Work out the finished part from the listing and answer in its coordinate system (mm). Round coordinates to 2 decimals unless told otherwise and drop trailing zeros. Order: outer loops, then holes, each group sorted by start corner. A loop starts at its lowest first (then second) coordinate and runs counter-clockwise, first axis right, second up. Notation, with made-up numbers: M -9,88 L 10,88 A30 cw 10,114 Z; hole C 32,-32.75 d4. An arc over 180 degrees is marked long. Return JSON: item names as keys, results as strings.
from build123d import *

# Parameters (mm, degrees)
SKETCH1_R           = 2.25
SKETCH1_R_2         = 2.5
SKETCH1_W           = 86
SKETCH1_H           = 86
BOSS_EXTRUDE1_DEPTH = 1
FILLET1_R           = 5
FILLET2_R           = 10


with BuildPart() as part:
    # Sketch1 → Boss-Extrude1 (new body)
    with BuildSketch(Plane(origin=(0, 0, 0), x_dir=(1, 0, 0), z_dir=(0, 1, 0))):
        Polygon((-70, -157.5), (447.5, -157.5), (447.5, -92.5), (82.5, -92.5), (82.5, 92.5), (447.5, 92.5), (447.5, 157.5), (-70, 157.5), align=None)
        with Locations(Location((-62.5, 100, 0), (0, 0, 270))):
            Circle(SKETCH1_R, mode=Mode.SUBTRACT)
        with Locations(Location((-62.5, -100, 0), (0, 0, 270))):
            Circle(SKETCH1_R, mode=Mode.SUBTRACT)
        with Locations(Location((-62.5, 150, 0), (0, 0, 270))):
            Circle(SKETCH1_R, mode=Mode.SUBTRACT)
        with Locations(Location((-62.5, -150, 0), (0, 0, 270))):
            Circle(SKETCH1_R, mode=Mode.SUBTRACT)
        with Locations(Location((62.5, -100, 0), (0, 0, 270))):
            Circle(SKETCH1_R, mode=Mode.SUBTRACT)
        with Locations(Location((62.5, -150, 0), (0, 0, 270))):
            Circle(SKETCH1_R, mode=Mode.SUBTRACT)
        with Locations(Location((62.5, 100, 0), (0, 0, 270))):
            Circle(SKETCH1_R, mode=Mode.SUBTRACT)
        with Locations(Location((62.5, 150, 0), (0, 0, 270))):
            Circle(SKETCH1_R, mode=Mode.SUBTRACT)
        with Locations(Location((187.5, -100, 0), (0, 0, 270))):
            Circle(SKETCH1_R, mode=Mode.SUBTRACT)
        with Locations(Location((187.5, -150, 0), (0, 0, 270))):
            Circle(SKETCH1_R, mode=Mode.SUBTRACT)
        with Locations(Location((187.5, 100, 0), (0, 0, 270))):
            Circle(SKETCH1_R, mode=Mode.SUBTRACT)
        with Locations(Location((187.5, 150, 0), (0, 0, 270))):
            Circle(SKETCH1_R, mode=Mode.SUBTRACT)
        with Locations(Location((312.5, -100, 0), (0, 0, 270))):
            Circle(SKETCH1_R, mode=Mode.SUBTRACT)
        with Locations(Location((312.5, -150, 0), (0, 0, 270))):
            Circle(SKETCH1_R, mode=Mode.SUBTRACT)
        with Locations(Location((312.5, 100, 0), (0, 0, 270))):
            Circle(SKETCH1_R, mode=Mode.SUBTRACT)
        with Locations(Location((312.5, 150, 0), (0, 0, 270))):
            Circle(SKETCH1_R, mode=Mode.SUBTRACT)
        with Locations(Location((437.5, -100, 0), (0, 0, 270))):
            Circle(SKETCH1_R, mode=Mode.SUBTRACT)
        with Locations(Location((437.5, -150, 0), (0, 0, 270))):
            Circle(SKETCH1_R, mode=Mode.SUBTRACT)
        with Locations(Location((437.5, 100, 0), (0, 0, 270))):
            Circle(SKETCH1_R, mode=Mode.SUBTRACT)
        with Locations(Location((437.5, 150, 0), (0, 0, 270))):
            Circle(SKETCH1_R, mode=Mode.SUBTRACT)
        with Locations(Location((-43, -73, 0), (0, 0, 270))):
            Circle(SKETCH1_R_2, mode=Mode.SUBTRACT)
        with Locations(Location((43, -73, 0), (0, 0, 270))):
            Circle(SKETCH1_R_2, mode=Mode.SUBTRACT)
        with Locations(Location((-43, 73, 0), (0, 0, 270))):
            Circle(SKETCH1_R_2, mode=Mode.SUBTRACT)
        with Locations(Location((43, 73, 0), (0, 0, 270))):
            Circle(SKETCH1_R_2, mode=Mode.SUBTRACT)
        with Locations(Location((262.5, 150, 0), (0, 0, 270))):
            Circle(SKETCH1_R, mode=Mode.SUBTRACT)
        with Locations(Location((262.5, 100, 0), (0, 0, 270))):
            Circle(SKETCH1_R, mode=Mode.SUBTRACT)
        with Locations(Location((262.5, -100, 0), (0, 0, 270))):
            Circle(SKETCH1_R, mode=Mode.SUBTRACT)
        with Locations(Location((262.5, -150, 0), (0, 0, 270))):
            Circle(SKETCH1_R, mode=Mode.SUBTRACT)
        Rectangle(SKETCH1_W, SKETCH1_H, mode=Mode.SUBTRACT)
    extrude(amount=BOSS_EXTRUDE1_DEPTH)

    # Fillet1
    fillet1_edges = [part.edges().sort_by_distance(p)[0] for p in [
        (447.5, 0.5, 92.5),
        (447.5, 0.5, 157.5),
        (-70, 0.5, 157.5),
        (-70, 0.5, -157.5),
        (447.5, 0.5, -157.5),
        (447.5, 0.5, -92.5),
    ]]
    fillet(fillet1_edges, radius=FILLET1_R)

    # Fillet2
    fillet2_edges = [part.edges().sort_by_distance(p)[0] for p in [
        (82.5, 0.5, -92.5),
        (82.5, 0.5, 92.5),
    ]]
    fillet(fillet2_edges, radius=FILLET2_R)


solid = part.part
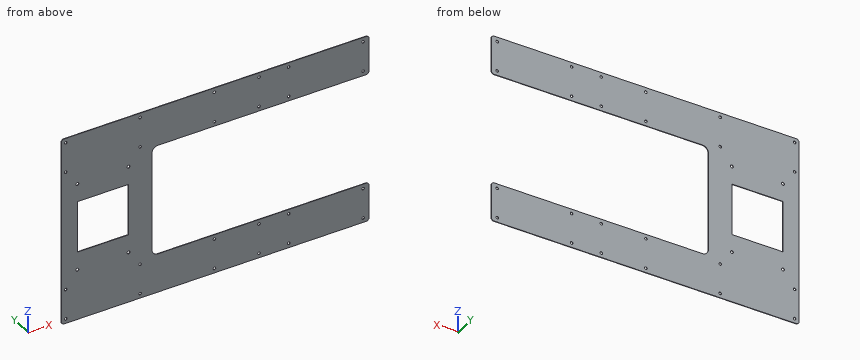
Item 1: Find section B-B (x = 142). Determine the outline of the cut face in (y, z).
Output:
{"outline": "M 0,-157.5 L 1,-157.5 L 1,-92.5 L 0,-92.5 Z; M 0,92.5 L 1,92.5 L 1,157.5 L 0,157.5 Z"}
Item 2: Consider line 1 along Z through (x, y) = (262.5, 0.55); line 2 along Z through (x, y) = (11.5, 0.35); line 3 along Z through (x, y) = (204.5, 0.55). Determine where each line is inside the solid, lowest interval first. Write a range as [from, to].
Output:
{"line 1": "z = [-157.5, -152.25], [-147.75, -102.25], [-97.75, -92.5], [92.5, 97.75], [102.25, 147.75], [152.25, 157.5]", "line 2": "z = [-157.5, -43], [43, 157.5]", "line 3": "z = [-157.5, -92.5], [92.5, 157.5]"}
Item 3: This flat-tipped pin is pushed along its axis until it touches: pin 1 (4 mm diameter, centred on x = -62.5, z = 150, fed in from -Y). Where does it stop, or does it pass through?
Output:
{"pin 1": "passes through"}
Item 4: Find section A-A (z = -16). Determine the outline of the cut face in (x, y).
Output:
{"outline": "M -70,0 L -43,0 L -43,1 L -70,1 Z; M 43,0 L 82.5,0 L 82.5,1 L 43,1 Z"}
Item 5: Find section C-C (y = 0.7). State how many separate pieces and enclosed holes the cut face has, plus the area to 3 significant figures.
Output:
{"separate pieces": "1", "enclosed holes": "29", "area": "87,600 mm^2"}
